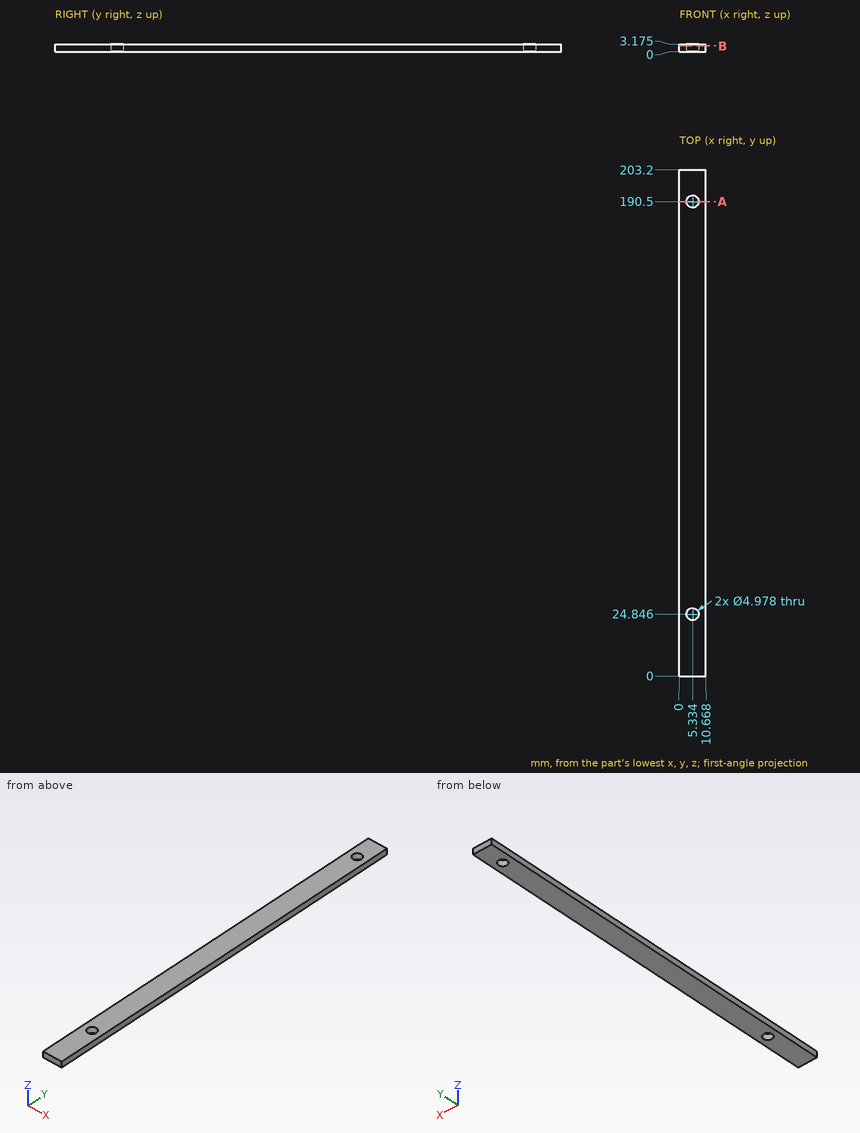
For this review, use the dimensioned drawing (mm, ordinates from the lowest corner) and the shaded views. Round coordinates to 2 decimals unless told otherwise and drop trailing zeros. Order: outer loops, then holes, each group sorted by start corner. A loop starts at its lowest first (then second) coordinate and runs counter-clockwise, first axis right, second up. Notation, with made-up numbers: M -9,-10 L 1,-10 A26 ccw 1,12 Z; hole C 74.25,47.5 d10. An arc over 180 degrees is marked long. Use a Markdown table: item, result.
1) Consider section B-B (z = 2.4). Write out the cut boundary in (x, y) (1 decimal).
Report:
| item | result |
|---|---|
| outline | M 0,0 L 10.7,0 L 10.7,203.2 L 0,203.2 Z; hole C 5.3,24.8 d5; hole C 5.3,190.5 d5 |
2) Consider section A-A (y = 190.5). Write out the cut boundary in (x, z) (1 decimal).
Report:
| item | result |
|---|---|
| outline | M 0,0 L 2.8,0 L 2.8,3.2 L 0,3.2 Z; M 7.8,0 L 10.7,0 L 10.7,3.2 L 7.8,3.2 Z |
3) Insertion check: pin 1 (6 mm diameter, centred on x = 6.5, y = 57.5, fed in from -Z). The pin has a flat end and moves straight along its axis. Give the tip position at first contact, or say it passes through.
Report:
| item | result |
|---|---|
| pin 1 | z = 0 |
4) Wall thickness on line 1 along Y through (x, z) = (5.5, 1.1); line 2 along X through (y, z) = (190.5, 0.75) (1 decimal); line 3 along Y through (x, z) = (6.25, 1.4) (1 decimal): over which ranges is each line inside the solid? List them lowest first. Write a range as [from, to].
Report:
| item | result |
|---|---|
| line 1 | [0, 22.36], [27.33, 188.02], [192.98, 203.2] |
| line 2 | [0, 2.8], [7.8, 10.7] |
| line 3 | [0, 22.5], [27.2, 188.2], [192.8, 203.2] |
